For this review, take the finished solid that the model builds, in its own axes (mm). Face numbers are marked on the shaded views. A direction names the side the tool comes from. Round coordinates to 2 decimals unless told otherwise and drop trailing zeros. Write each loop counter-clockwise with the first axis right and the second up, starting at its lowest first coordinate (ties: lowest second). Pieces come first, ordered by that corner, then holes. Notation, with made-up numbers: (-37.75, 21) -> (-31.75, 21) arc R10 ccw to (-31.75, 33) -> close; hole circle Ø3 at (79, 33). An arc over 180 degrees is marked (long way). Answer as CSV lines item,"result". Start each with the question number.
Item 1: Wall thickness on probe 1 along X at (y, z) = (-25, 13); probe 2 along Y at (x, z) = (0, -15.5); probe 3 along Z at (x, y) = (22.5, -6): over which ranges is each line inside the solid? List them lowest first. Write a range as from..to.
Item 2: For pin 1 Ø11 at (x, z) = (-14.5, 10.5) entering from +Y; pin 2 Ø22.5 at (x, y) = (0, -25) entering from +Z; pin 3 Ø6 at (x, z) = (-23.5, -13.5) entering from +Y; pin 4 Ø1 at (x, z) = (-6, -15) entering from -Y, all flat-tipped, find the tip position at first contact; note any pin that passes through.
Item 3: Take a section at C-C on y = -14. Give the boundary of the cut face in (x, z).
Item 4: Take a section at D-D on x = -2. Give the boundary of the cut face in (y, z), then the cut area to 3 significant figures.
Item 5: Take a section at B-B on y = 82. Give the boundary of the cut face in (x, z).
Item 6: Mouldability with a two-part tool opening along Z and no side actions: class the marked faces 5, 6 and 7 as +Z half, -Z half, draft (parallel to the pull), parting line (faces both ways), or undercut.
Item 7: Machinability: for the marked faces 1, 2, 3 and 4, which of the approach directions +Z, -Z, +X, -X, +Y, -Y give a long, thin tool a straight path to every point of the face, cutting with its end or side? Answer none if there is none.
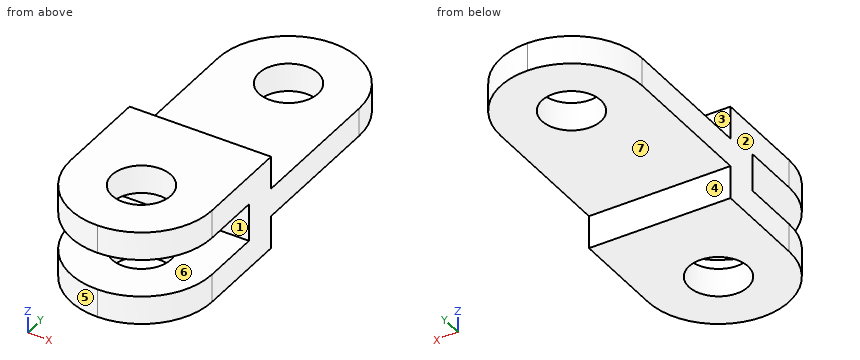
```python
from build123d import *

# Parameters (mm, degrees)
BOSS_EXTRUDE1_DEPTH     = 30
FILLET1_R               = 30
CUT_EXTRUDE1_DEPTH      = 117.297033496
CUT_EXTRUDE1_DEPTH_BACK = 117.297033496
SKETCH3_R               = 12.5


with BuildPart() as part:
    # Sketch1 → Boss-Extrude1 (new, symmetric)
    with BuildSketch(Plane.YZ):
        Polygon((0, -8), (0, 8), (-55, 8), (-55, 20), (15, 20), (15, 6), (105, 6), (105, -6), (15, -6), (15, -20), (-55, -20), (-55, -8), align=None)
    extrude(amount=BOSS_EXTRUDE1_DEPTH, both=True)

    # Fillet1
    fillet1_edges = [part.edges().sort_by_distance(p)[0] for p in [
        (-30, 105, 0),
        (30, 105, 0),
        (30, -55, -14),
        (-30, -55, -14),
        (-30, -55, 14),
        (30, -55, 14),
    ]]
    fillet(fillet1_edges, radius=FILLET1_R - 0.0001)  # a hair under: the kernel refuses the full size

    # Sketch3 → Cut-Extrude1 (cut, two sides: drawn at the far end of the back side and taken through both)
    with BuildSketch(Plane.XY.offset(20).offset(-CUT_EXTRUDE1_DEPTH_BACK)):
        with Locations((0, -25)):
            Circle(SKETCH3_R)
        with Locations((0, 75)):
            Circle(SKETCH3_R)
    extrude(amount=CUT_EXTRUDE1_DEPTH + CUT_EXTRUDE1_DEPTH_BACK, mode=Mode.SUBTRACT)


solid = part.part
```
Output values:
1,probe 1,"x = -30..-12.5, 12.5..30"
1,probe 2,"y = -55..-37.5, -12.5..15"
1,probe 3,"z = -20..-8, 8..20"
2,pin 1,"stops at y = 102.78"
2,pin 2,"passes through"
2,pin 3,"stops at y = 15"
2,pin 4,"stops at y = -54.49"
3,outline,"(-30, -20) -> (-5.94, -20) -> (-5.94, -8) -> (-30, -8) -> close; (-30, 8) -> (-5.94, 8) -> (-5.94, 20) -> (-30, 20) -> close; (5.94, -20) -> (30, -20) -> (30, -8) -> (5.94, -8) -> close; (5.94, 8) -> (30, 8) -> (30, 20) -> (5.94, 20) -> close"
4,outline,"(-54.93, -20) -> (-37.34, -20) -> (-37.34, -8) -> (-54.93, -8) -> close; (-54.93, 8) -> (-37.34, 8) -> (-37.34, 20) -> (-54.93, 20) -> close; (-12.66, -20) -> (15, -20) -> (15, -6) -> (62.66, -6) -> (62.66, 6) -> (15, 6) -> (15, 20) -> (-12.66, 20) -> (-12.66, 8) -> (0, 8) -> (0, -8) -> (-12.66, -8) -> close; (87.34, -6) -> (104.93, -6) -> (104.93, 6) -> (87.34, 6) -> close"
4,area,"2,110 mm^2"
5,outline,"(-29.17, -6) -> (-10.36, -6) -> (-10.36, 6) -> (-29.17, 6) -> close; (10.36, -6) -> (29.17, -6) -> (29.17, 6) -> (10.36, 6) -> close"
6,face 5,"draft"
6,face 6,"undercut"
6,face 7,"-Z half"
7,face 1,"+X, -X, -Y"
7,face 2,"+Z, -Z, -X, +Y, -Y"
7,face 3,"+Z, +X, -X, +Y"
7,face 4,"-Z, +X, -X, +Y"
